Design review of the part shown in the three views and the two pictorial views. Dimensions are in mm from the part's minimum x, y and z. A direction names the side the tool comes from. Round coordinates to 2 decimals unless told otherwise and drop trailing zeros. Order: outer loops, then holes, each group sorted by start corner. A loop starts at its lowest first (then second) coordinate and runs counter-clockwise, first axis right, second up. Notation, with made-up numbers: (22, 35) - (42, 35) arc R20 cw to (42, 46) - close; hole circle Ø7 at (68, 28.25). An arc over 180 degrees is marked (long way). One line per question, with ' | ' between items. Start each with the question number.
Item 1: Add section B-B on x = 23. State the section outline as (y, z) points.
Item 2: Add section D-D on x = 9. State the section outline as (y, z) points, and give its area (3 significant figures).
Item 3: Draft analysis for pull direction Z (two halves, no side actions). For the marked faces 1, 2 and 3, state which applies: +Z half, -Z half, draft (parallel to the pull), parting line (faces both ways), or undercut.
Item 4: Add section A-A on y = 16. State the section outline as (x, z) points, and give its area (3 significant figures).
Item 5: Tool access review of the marked faces 4, 5, 6, 7 and 8: name each direction out of +Z, -Z, +X, -X, +Y, -Y from which nothing blocks a thin tool from reaching the whole face with its end or side.
Item 6: For L1, parallel to Y at x = 23, z = 45.5; L2, parallel to Z at x = 22, y = 41; L3, parallel to Y at x = 6, z = 28, list the stretches that pass through material, from the lowest coordinate up. Write a range as [from, to].
Item 7: Add section C-C on z = 43. State the section outline as (x, y) points.
Item 8: Insertion check: pin 1 Ø18 at (x, y) = (12.5, 33) entering from +Z; pin 2 Ø11 at (x, y) = (30, 27.5) entering from -Z; pin 3 Ø3.5 at (x, z) = (27.5, 57) entering from +Y. Each pin has a flat end and moves straight along its axis. Give the tip position at first contact, or say it passes through.
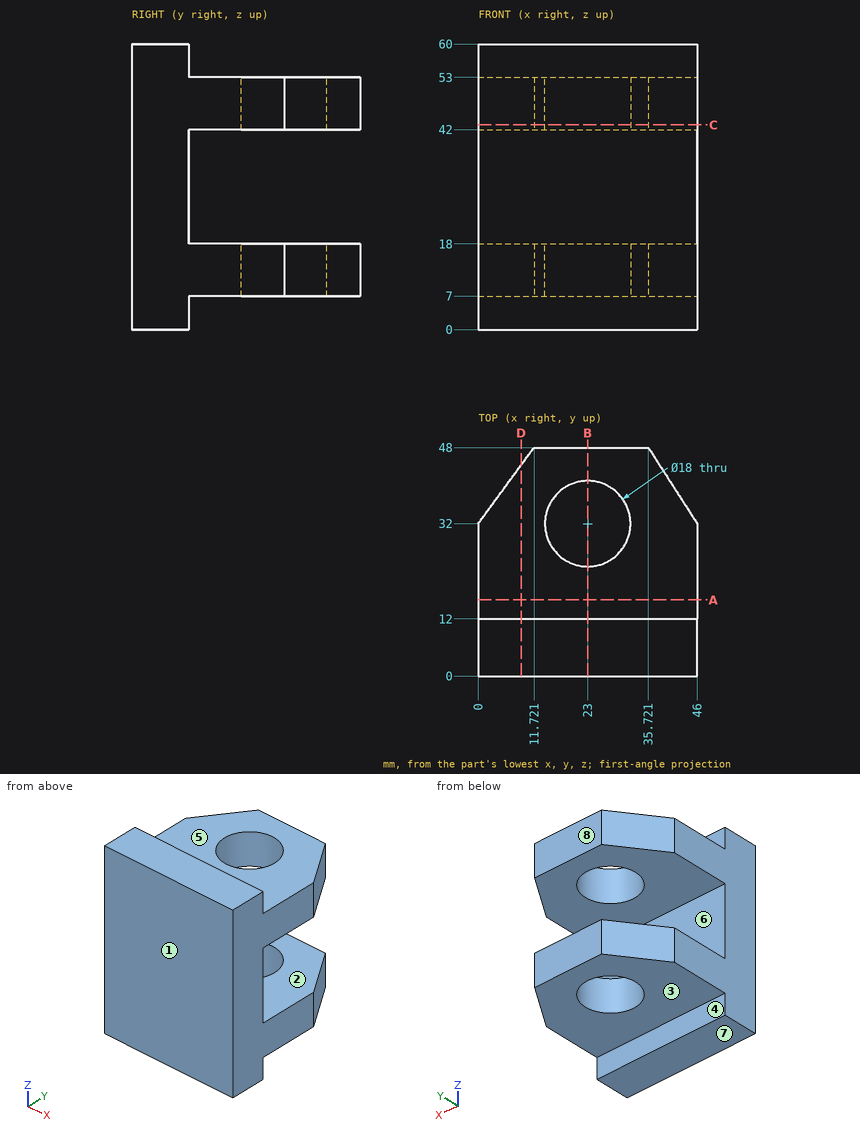
Determined:
1) outline: (0, 0) - (12, 0) - (12, 7) - (23, 7) - (23, 18) - (12, 18) - (12, 42) - (23, 42) - (23, 53) - (12, 53) - (12, 60) - (0, 60) - close; (41, 7) - (48, 7) - (48, 18) - (41, 18) - close; (41, 42) - (48, 42) - (48, 53) - (41, 53) - close
2) outline: (0, 0) - (12, 0) - (12, 7) - (44.29, 7) - (44.29, 18) - (12, 18) - (12, 42) - (44.29, 42) - (44.29, 53) - (12, 53) - (12, 60) - (0, 60) - close | area: 1,430 mm2
3) face 1: draft | face 2: undercut | face 3: -Z half
4) outline: (0, 7) - (46, 7) - (46, 18) - (0, 18) - close; (0, 42) - (46, 42) - (46, 53) - (0, 53) - close | area: 1,010 mm2
5) face 4: -Z, +X, -X, +Y | face 5: +Z, +X, -X, +Y | face 6: +X, -X, +Y | face 7: -Z, +X, -X, +Y, -Y | face 8: +Z, -Z, +X, -X, +Y
6) L1: [0, 23], [41, 48] | L2: [7, 18], [42, 53] | L3: [0, 12]
7) outline: (0, 0) - (46, 0) - (46, 32) - (35.72, 48) - (11.72, 48) - (0, 32) - close; hole circle Ø18 at (23, 32)
8) pin 1: z = 53 | pin 2: z = 7 | pin 3: y = 12
